```python
from build123d import *

# Parameters (mm, degrees)
F0_W     = 161.15
F0_H     = 17.5
F1_DEPTH = 2.4
F2_W     = 161.15
F2_H     = 2.4
F3_DEPTH = 0.6
F4_W     = 161.15
F4_H     = 2.4
F5_DEPTH = 0.6
F6_W     = 2.4
F6_H     = 12.7
F7_DEPTH = 0.6


with BuildPart() as f1:
    # F0 (on Top) → F1 (new body)
    with BuildSketch(Plane.XY):
        with Locations((74.009652, 20.676134)):
            Rectangle(F0_W, F0_H)
    extrude(amount=F1_DEPTH)

    # F2 (on face) → F3 (join)
    with BuildSketch(Plane(origin=(0, 0, 0), x_dir=(1, 0, 0), z_dir=(0, 0, -1))):
        with Locations((74.009652, -28.226134)):
            Rectangle(F2_W, F2_H)
    extrude(amount=F3_DEPTH)

    # F4 (on face) → F5 (join)
    with BuildSketch(Plane(origin=(0, 0, 0), x_dir=(1, 0, 0), z_dir=(0, 0, -1))):
        with Locations((74.009652, -13.126134)):
            Rectangle(F4_W, F4_H)
    extrude(amount=F5_DEPTH)

    # F6 (on face) → F7 (join)
    with BuildSketch(Plane(origin=(0, 0, 0), x_dir=(1, 0, 0), z_dir=(0, 0, -1))):
        with Locations((-5.365348, -20.676134)):
            Rectangle(F6_W, F6_H)
    extrude(amount=F7_DEPTH)


solid = f1.part
```
Could you check a few things on this model? Use its own coordinates, in mm. A direction names the side the tool comes from. Coordinates: 2 decimals unless noted, no trailing zeros. Order: outer loops, then holes, each group sorted by start corner. A loop starts at its lowest first (then second) coordinate and runs counter-clockwise, first axis right, second up. Notation, with made-up numbers: M 54,74 L 68,74 A16 cw 68,91 Z; hole C -5,42 d3. An arc over 180 degrees is marked long. Use a Markdown table: item, result. Add a question column.
Q1. If I drill on L1, parallel to Y at x = 9, z = -0.2; L2, parallel to X at y = 16.75, z = -0.4; L3, parallel to Z at x = 115, y = 24.5, over which ranges is the centre line in solid material (lowest first)?
Q2. We'd pull the mould along X, two halves only. Please class faces 1 (the flat face through (73, 21, 2.4)), 2 (the flat face through (-6.565, 21, 1)), 3 (the flat face through (154.585, 21, 1)): pulls with the +X half, pulls with the -X half, needs draft (parallel to the pull), parting line crosses it, or undercut.
Q3. I want a section at B-B on y = 23.5. List the corners of the cut face in (x, z) for me.
Q4. I'm going to push a flat-ended pin straight in: pin 1 (4 mm diameter, centred on x = 77, y = 22.5, fed in from -Z). Where does the tip first touch, or does it pass through?
Q5. I want a section at A-A on x = 129. List the corners of the cut face in (y, z) for me, then the cut area to 3 significant figures.
Q6. Which directions (+Z, -Z, +X, -X, +Y, -Y) give clear straight access to the entire face, cutting with the end or side of a thin tool? Please do faces 4 (the flat face through (74, 14, -0.6)), 5 (the flat face through (74, 21, 0)).
Checked values:
| question | item | result |
|---|---|---|
| 1 | L1 | 11.93 to 14.33, 27.03 to 29.43 |
| 1 | L2 | -6.57 to -4.17 |
| 1 | L3 | 0 to 2.4 |
| 2 | face 1 | needs draft |
| 2 | face 2 | pulls with the -X half |
| 2 | face 3 | pulls with the +X half |
| 3 | outline | M -6.57,-0.6 L -4.17,-0.6 L -4.17,0 L 154.58,0 L 154.58,2.4 L -6.57,2.4 Z |
| 4 | pin 1 | z = 0 |
| 5 | outline | M 11.93,-0.6 L 14.33,-0.6 L 14.33,0 L 27.03,0 L 27.03,-0.6 L 29.43,-0.6 L 29.43,2.4 L 11.93,2.4 Z |
| 5 | area | 44.9 mm² |
| 6 | face 4 | -Z, +X, -X, +Y, -Y |
| 6 | face 5 | -Z, +X |
